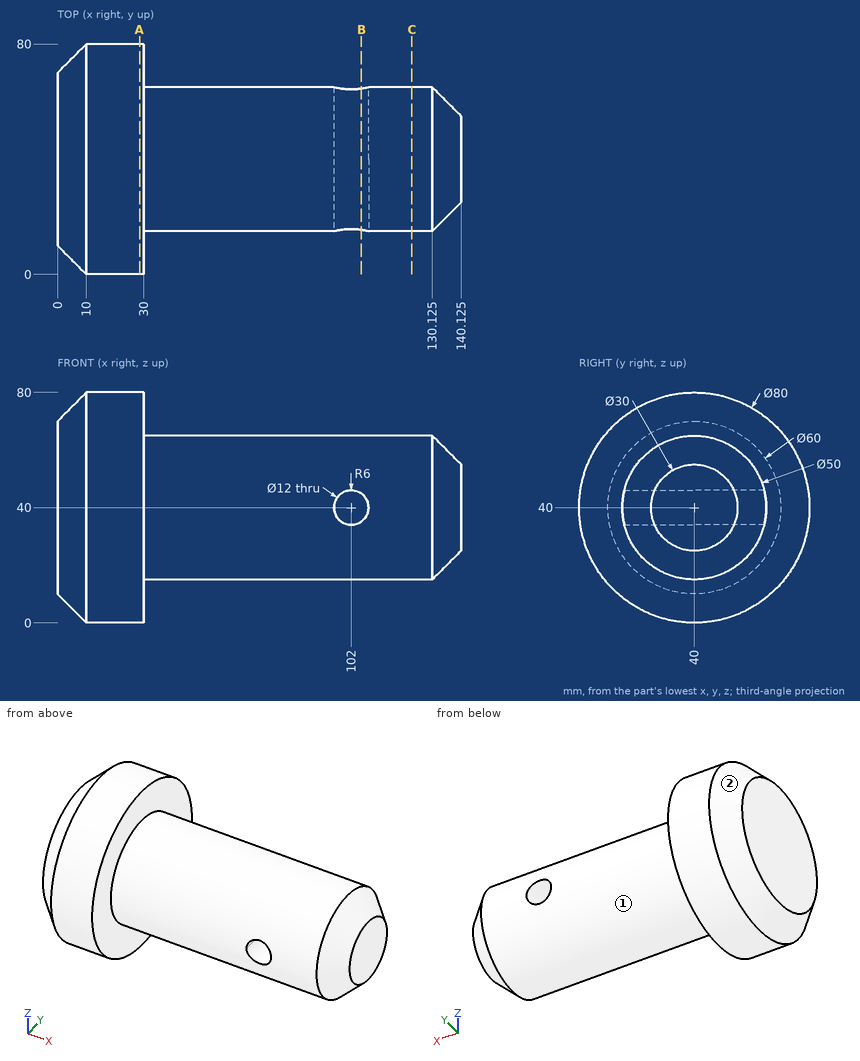
Print and shaded views of the part. All mm, measured from the part's lowest x, y and z. A direction names the side the tool comes from. Coordinates: 2 decimals unless noted, no trailing zeros. Order: outer loops, then holes, each group sorted by start corner. A loop starts at its lowest first (then second) coordinate and runs counter-clockwise, first axis right, second up. Notation, with made-up numbers: (84.25, 60) -> (127.25, 60) arc R14 cw to (127.25, 72) -> close; hole circle Ø7 at (-29, 39.25). An arc over 180 degrees is marked (long way). Answer as a JSON object with one key per item and string values. Group by question number.
1) Flat gauge pins, fed straight in: pin 1 (6 mm diameter, centred on y = 26, z = 72, fed in from +X); pin 2 (12 mm diameter, centred on y = 34.5, z = 15, fed in from +X); pin 3 (14 mm diameter, centred on x = 102, z = 40, fed in from +Y); pin 4 (6 mm diameter, centred on y = 25.5, z = 57.5, fed in from -X). Where does each tip first touch, or does it go through?
2) Cut at A-A, the plane x = 28.5. Write the cut outline in (y, z), then the cut area to 3 significant figures.
3) Cut at C-C, the plane x = 123. Write the cut outline in (y, z), then the cut area to 3 significant figures.
4) Drill centre lines: L1, parallel to X at y = 54, z = 40 (1 decimal); L2, parallel to X at y = 52, z = 16; L3, parallel to X at y = 59.75, z = 40 (1 decimal). Where is each one in solid material? Low to high.
5) Cut at B-B, the plane x = 105.5. Write the cut outline in (y, z).
6) Which spindle directions (+Z, -Z, +X, -X, +Y, -Y) get a long thin tool onto all of the face, cutting with end or side? Do the marked faces 1 and 2. Say none if no direction does.
Check values:
{
 "1": {"pin 1": "stops at x = 30", "pin 2": "stops at x = 135.53", "pin 3": "stops at y = 65", "pin 4": "stops at x = 0"},
 "2": {"outline": "circle Ø80 at (40, 40)", "area": "5,030 mm²"},
 "3": {"outline": "circle Ø50 at (40, 40)", "area": "1,960 mm²"},
 "4": {"L1": "x = 0 to 96, 108 to 140.1", "L2": "x = 0 to 30", "L3": "x = 0 to 96, 108 to 135.4"},
 "5": {"outline": "(15.48, 35.13) arc R25 ccw to (64.52, 35.13) -> close; (15.48, 44.87) -> (64.52, 44.87) arc R25 ccw to start"},
 "6": {"face 1": "+X", "face 2": "-X"}
}
